from build123d import *

# Parameters (mm, degrees)
BOSS_EXTRUDE1_DEPTH = 4.2
SKETCH2_W           = 62
SKETCH2_H           = 40
BOSS_EXTRUDE2_DEPTH = 1.5
FILLET1_R           = 0.5


with BuildPart() as part:
    # Sketch1 → Boss-Extrude1 (new body)
    with BuildSketch(Plane.XY):
        with BuildLine():
            Line((-5, 73.5), (-34.5, 73.5))
            Line((-34.5, 73.5), (-34.5, 26.5))
            Line((-34.5, 26.5), (34.5, 26.5))
            Line((34.5, 26.5), (34.5, 73.5))
            Line((34.5, 73.5), (5, 73.5))
            Line((5, 73.5), (5, 71))
            Line((5, 71), (31.24600638, 71))
            ThreePointArc((31.24600638, 71), (32.245433101, 72.825781164), (33.85, 71.5))
            ThreePointArc((33.85, 71.5), (33.25746287, 70.382525168), (32, 70.24600638))
            Line((32, 70.24600638), (32, 29.75399362))
            ThreePointArc((32, 29.75399362), (33.25746287, 29.617474832), (33.85, 28.5))
            ThreePointArc((33.85, 28.5), (32.245433101, 27.174218836), (31.24600638, 29))
            Line((31.24600638, 29), (-31.24600638, 29))
            ThreePointArc((-31.24600638, 29), (-31.174218836, 28.754566899), (-31.15, 28.5))
            ThreePointArc((-31.15, 28.5), (-33.617474832, 27.74253713), (-32, 29.75399362))
            Line((-32, 29.75399362), (-32, 70.24600638))
            ThreePointArc((-32, 70.24600638), (-33.617474832, 72.25746287), (-31.15, 71.5))
            ThreePointArc((-31.15, 71.5), (-31.174218836, 71.245433101), (-31.24600638, 71))
            Line((-31.24600638, 71), (-5, 71))
            Line((-5, 71), (-5, 73.5))
        make_face()
    extrude(amount=BOSS_EXTRUDE1_DEPTH)

    # Sketch2 → Boss-Extrude2 (add)
    # profile 1 of 2: a face of its own
    with BuildSketch(Plane.XY.offset(4.2)):
        with BuildLine():
            Line((31.24600638, 29), (-31.24600638, 29))
            ThreePointArc((-31.24600638, 29), (-33.454594155, 27.545405845), (-32, 29.75399362))
            Line((-32, 29.75399362), (-32, 70.24600638))
            ThreePointArc((-32, 70.24600638), (-33.454594155, 72.454594155), (-31.24600638, 71))
            Line((-31.24600638, 71), (-5, 71))
            Line((-5, 71), (-5, 73.5))
            Line((-5, 73.5), (-34.5, 73.5))
            Line((-34.5, 73.5), (-34.5, 26.5))
            Line((-34.5, 26.5), (34.5, 26.5))
            Line((34.5, 26.5), (34.5, 73.5))
            Line((34.5, 73.5), (5, 73.5))
            Line((5, 73.5), (5, 71))
            Line((5, 71), (31.24600638, 71))
            ThreePointArc((31.24600638, 71), (33.454594155, 72.454594155), (32, 70.24600638))
            Line((32, 70.24600638), (32, 29.75399362))
            ThreePointArc((32, 29.75399362), (33.454594155, 27.545405845), (31.24600638, 29))
        make_face()
    # profile 2 of 2: a face of its own
    with BuildSketch(Plane.XY.offset(4.2)):
        with BuildLine():
            Line((5, 71), (5, 73.5))
            Line((5, 73.5), (-5, 73.5))
            Line((-5, 73.5), (-5, 71))
            Line((-5, 71), (-31.24600638, 71))
            ThreePointArc((-31.24600638, 71), (-31.545405845, 70.545405845), (-32, 70.24600638))
            Line((-32, 70.24600638), (-32, 29.75399362))
            ThreePointArc((-32, 29.75399362), (-31.545405845, 29.454594155), (-31.24600638, 29))
            Line((-31.24600638, 29), (31.24600638, 29))
            ThreePointArc((31.24600638, 29), (31.545405845, 29.454594155), (32, 29.75399362))
            Line((32, 29.75399362), (32, 70.24600638))
            ThreePointArc((32, 70.24600638), (31.545405845, 70.545405845), (31.24600638, 71))
            Line((31.24600638, 71), (5, 71))
        make_face()
        with Locations((0, 50)):
            Rectangle(SKETCH2_W, SKETCH2_H, mode=Mode.SUBTRACT)
    extrude(amount=BOSS_EXTRUDE2_DEPTH)

    # Fillet1
    fillet1_edges = [part.edges().sort_by_distance(p)[0] for p in [
        (34.5, 73.5, 2.85),
        (34.5, 26.5, 2.85),
        (-34.5, 26.5, 2.85),
        (-34.5, 73.5, 2.85),
        (-31, 50, 5.7),
        (0, 30, 5.7),
        (34.5, 50, 5.7),
        (0, 73.5, 5.7),
        (-34.5, 50, 5.7),
        (0, 26.5, 5.7),
        (0, 70, 5.7),
        (31, 50, 5.7),
    ]]
    fillet(fillet1_edges, radius=FILLET1_R)


solid = part.part
Geometry check sheet. Reference: the model listing, model coordinates, mm. A direction names the side the tool comes from. Give positions to 0.01 mm unless a question says otherwise; leave off trailing zeros. Order: outer loops, then holes, each group sorted by start corner. A loop starts at its lowest first (then second) coordinate and runs counter-clockwise, first axis right, second up.
1) Material ranges on probe 1 along Y at (x, z) = (32.5, 1.4); probe 2 along X at (y, z) = (28.5, 5.1); probe 3 along X at (y, z) = (71.5, 1.2), recorded low to high.
Results are:
probe 1: y = 26.5 to 27.15, 29.85 to 70.15, 72.85 to 73.5
probe 2: x = -34.5 to -33.85, -31.15 to 31.15, 33.85 to 34.5
probe 3: x = -34.5 to -33.85, -31.15 to -5, 5 to 31.15, 33.85 to 34.5
2) Cross-section at D-D (x = 20.5). Record the boundary of the cut face in (y, z).
Results are:
outline: (26.5, 0) - (29, 0) - (29, 4.2) - (30, 4.2) - (30, 5.2) arc R0.5 ccw to (29.5, 5.7) - (27, 5.7) arc R0.5 ccw to (26.5, 5.2) - close; (70, 4.2) - (71, 4.2) - (71, 0) - (73.5, 0) - (73.5, 5.2) arc R0.5 ccw to (73, 5.7) - (70.5, 5.7) arc R0.5 ccw to (70, 5.2) - close
3) Cross-section at C-C (z = 1.7). Record the boundary of the cut face in (x, y), then the cut area to 3 significant figures.
Results are:
outline: (-34.5, 27) arc R0.5 ccw to (-34, 26.5) - (34, 26.5) arc R0.5 ccw to (34.5, 27) - (34.5, 73) arc R0.5 ccw to (34, 73.5) - (5, 73.5) - (5, 71) - (31.25, 71) arc R1.35 cw (long way) to (32, 70.25) - (32, 29.75) arc R1.35 cw (long way) to (31.25, 29) - (-31.25, 29) arc R1.35 cw (long way) to (-32, 29.75) - (-32, 70.25) arc R1.35 cw (long way) to (-31.25, 71) - (-5, 71) - (-5, 73.5) - (-34, 73.5) arc R0.5 ccw to (-34.5, 73) - close
area: 508 mm2
4) Cross-section at B-B (y = 43). Record the boundary of the cut face in (x, z).
Results are:
outline: (-34.5, 0) - (-32, 0) - (-32, 4.2) - (-31, 4.2) - (-31, 5.2) arc R0.5 ccw to (-31.5, 5.7) - (-34, 5.7) arc R0.5 ccw to (-34.5, 5.2) - close; (31, 4.2) - (32, 4.2) - (32, 0) - (34.5, 0) - (34.5, 5.2) arc R0.5 ccw to (34, 5.7) - (31.5, 5.7) arc R0.5 ccw to (31, 5.2) - close
5) Cross-section at A-A (x = 3.5). Record the boundary of the cut face in (y, z), then the cut area to 3 significant figures.
Results are:
outline: (26.5, 0) - (29, 0) - (29, 4.2) - (30, 4.2) - (30, 5.2) arc R0.5 ccw to (29.5, 5.7) - (27, 5.7) arc R0.5 ccw to (26.5, 5.2) - close; (70, 4.2) - (73.5, 4.2) - (73.5, 5.2) arc R0.5 ccw to (73, 5.7) - (70.5, 5.7) arc R0.5 ccw to (70, 5.2) - close
area: 20.8 mm2
6) Tool access check on faces 1 (the flat face through (-34.5, 50, 3)), 2 (the flat face through (-5, 72, 2)), 3 (the flat face through (-32, 50, 2)). Record the directions out of +Z, -Z, +X, -X, +Y, -Y that give a thin tool (end or side, any length) a straight path to the whole face; none if there is none.
Results are:
face 1: +Z, -Z, -X, +Y, -Y
face 2: -Z, +Y
face 3: -Z
7) Draft check along X on faces 4 (the flat face through (34.5, 50, 3)), 5 (the flat face through (5, 72, 2)), 6 (the flat face through (0, 71, 5.7)), 7 (the flat face through (-18, 71, 2)). Enter one of: released by +X, released by -X, zero draft, split by the parting line, or undercut.
Results are:
face 4: released by +X
face 5: undercut
face 6: zero draft
face 7: undercut
8) Gauge pin test, flat end, axial feed: pin 1 (1.3 mm diameter, centred on x = 3.5, z = 2, fed in from +Y). Record the tip position at first contact, or that the pin passes through.
Results are:
pin 1: stops at y = 29
